from build123d import *

# Parameters (mm, degrees)
PCB_DIMENSION_R     = 0.6
PCB_DIMENSION_R_2   = 10
BOSS_EXTRUDE1_DEPTH = 1


with BuildPart() as part:
    # PCB dimension → Boss-Extrude1 (new body)
    with BuildSketch(Plane.XY):
        with BuildLine():
            Line((-1, 27.481812167), (-1, 28.981812167))
            Line((-1, 28.981812167), (1, 28.981812167))
            Line((1, 28.981812167), (1, 27.481812167))
            ThreePointArc((1, 27.481812167), (0, -27.5), (-1, 27.481812167))
        make_face()
        with Locations((15, 0)):
            Circle(PCB_DIMENSION_R, mode=Mode.SUBTRACT)
        with Locations((14.564127261, -3.589734964)):
            Circle(PCB_DIMENSION_R, mode=Mode.SUBTRACT)
        with Locations((13.281840385, -6.970847581)):
            Circle(PCB_DIMENSION_R, mode=Mode.SUBTRACT)
        with Locations((11.227661223, -9.946839874)):
            Circle(PCB_DIMENSION_R, mode=Mode.SUBTRACT)
        with Locations((8.520971201, -12.344757988)):
            Circle(PCB_DIMENSION_R, mode=Mode.SUBTRACT)
        with Locations((5.319073306, -14.02524364)):
            Circle(PCB_DIMENSION_R, mode=Mode.SUBTRACT)
        with Locations((1.808050204, -14.890633111)):
            Circle(PCB_DIMENSION_R, mode=Mode.SUBTRACT)
        with Locations((-1.808050204, -14.890633111)):
            Circle(PCB_DIMENSION_R, mode=Mode.SUBTRACT)
        with Locations((-5.319073306, -14.02524364)):
            Circle(PCB_DIMENSION_R, mode=Mode.SUBTRACT)
        with Locations((-8.520971201, -12.344757988)):
            Circle(PCB_DIMENSION_R, mode=Mode.SUBTRACT)
        with Locations((-11.227661223, -9.946839874)):
            Circle(PCB_DIMENSION_R, mode=Mode.SUBTRACT)
        with Locations((-13.281840385, -6.970847581)):
            Circle(PCB_DIMENSION_R, mode=Mode.SUBTRACT)
        with Locations((-14.564127261, -3.589734964)):
            Circle(PCB_DIMENSION_R, mode=Mode.SUBTRACT)
        with Locations((-15, 0)):
            Circle(PCB_DIMENSION_R, mode=Mode.SUBTRACT)
        with Locations((-14.564127261, 3.589734964)):
            Circle(PCB_DIMENSION_R, mode=Mode.SUBTRACT)
        with Locations((-13.281840385, 6.970847581)):
            Circle(PCB_DIMENSION_R, mode=Mode.SUBTRACT)
        with Locations((-11.227661223, 9.946839874)):
            Circle(PCB_DIMENSION_R, mode=Mode.SUBTRACT)
        with Locations((-8.520971201, 12.344757988)):
            Circle(PCB_DIMENSION_R, mode=Mode.SUBTRACT)
        with Locations((-5.319073306, 14.02524364)):
            Circle(PCB_DIMENSION_R, mode=Mode.SUBTRACT)
        with Locations((-1.808050204, 14.890633111)):
            Circle(PCB_DIMENSION_R, mode=Mode.SUBTRACT)
        with Locations((1.808050204, 14.890633111)):
            Circle(PCB_DIMENSION_R, mode=Mode.SUBTRACT)
        with Locations((5.319073306, 14.02524364)):
            Circle(PCB_DIMENSION_R, mode=Mode.SUBTRACT)
        with Locations((8.520971201, 12.344757988)):
            Circle(PCB_DIMENSION_R, mode=Mode.SUBTRACT)
        with Locations((11.227661223, 9.946839874)):
            Circle(PCB_DIMENSION_R, mode=Mode.SUBTRACT)
        with Locations((13.281840385, 6.970847581)):
            Circle(PCB_DIMENSION_R, mode=Mode.SUBTRACT)
        with Locations((14.564127261, 3.589734964)):
            Circle(PCB_DIMENSION_R, mode=Mode.SUBTRACT)
        Circle(PCB_DIMENSION_R_2, mode=Mode.SUBTRACT)
    extrude(amount=BOSS_EXTRUDE1_DEPTH)


solid = part.part
Source: CAD feature listing. Evaluate the final solid. Frame: model axes, mm. Coordinates: 2 decimals unless noted, no trailing zeros. Order: outer loops, then holes, each group sorted by start corner. A loop starts at its lowest first (then second) coordinate and runs counter-clockwise, first axis right, second up. Notation, with made-up numbers: M 3,-39 L 47,-39 A30 cw 47,-1 Z; hole C 54.5,-5 d2. An arc over 180 degrees is marked long. Write each question's results on one line, items separated by ' | '. Start each with the question number.
1. Section A-A, the plane x = 0. Return the cut outline in (y, z), then the cut area to 3 significant figures.
2. Material intervals for L1, parallel to X at y = -7, z = 0.35; L2, parallel to X at y = 4, z = 0.7; L3, parallel to Y at x = 15, z = 0.5, sorted ascending.
3. Draft query along X for faces 1 (the face through (5.19, 13.44, 0.49)), 2 (the face through (0, -11, 0)), 3 (the face through (1.195, -27.474, 0.493)). Return one class per face: +X half, -X half, draft (parallel to the pull), parting line (faces both ways), or undercut.
4. Section D-D, the plane y = 16.5. Return the cut outline in (x, z), then the cut area to 3 significant figures.
5. Section B-B, the plane y = -1.5. Return the cut outline in (x, z).
6. Pin query (flat end, axial travel): pin 1 (1 mm diameter, centred on x = 11.23, y = 9.95, fed in from +Z). Return the tip coordinate at first contact, or that it passes through.
7. Section C-C, the plane z = 0.3. State how many separate pieces and enclosed holes the cut face has, then the cut area to 3 significant figures.
Solution:
1) outline: M -27.5,0 L -10,0 L -10,1 L -27.5,1 Z; M 10,0 L 28.98,0 L 28.98,1 L 10,1 Z | area: 36.5 mm²
2) L1: -26.59 to -13.88, -12.68 to -7.14, 7.14 to 12.68, 13.88 to 26.59 | L2: -27.21 to -15, -14.13 to -9.17, 9.17 to 14.13, 15 to 27.21 | L3: -23.05 to -4, -3.18 to -0.6, 0.6 to 3.18, 4 to 23.05
3) face 1: undercut | face 2: draft | face 3: parting line
4) outline: M -22,0 L 22,0 L 22,1 L -22,1 Z | area: 44.0 mm²
5) outline: M -27.46,0 L -9.89,0 L -9.89,1 L -27.46,1 Z; M 9.89,0 L 27.46,0 L 27.46,1 L 9.89,1 Z
6) pin 1: through
7) separate pieces: 1 | enclosed holes: 27 | area: 2,040 mm²
